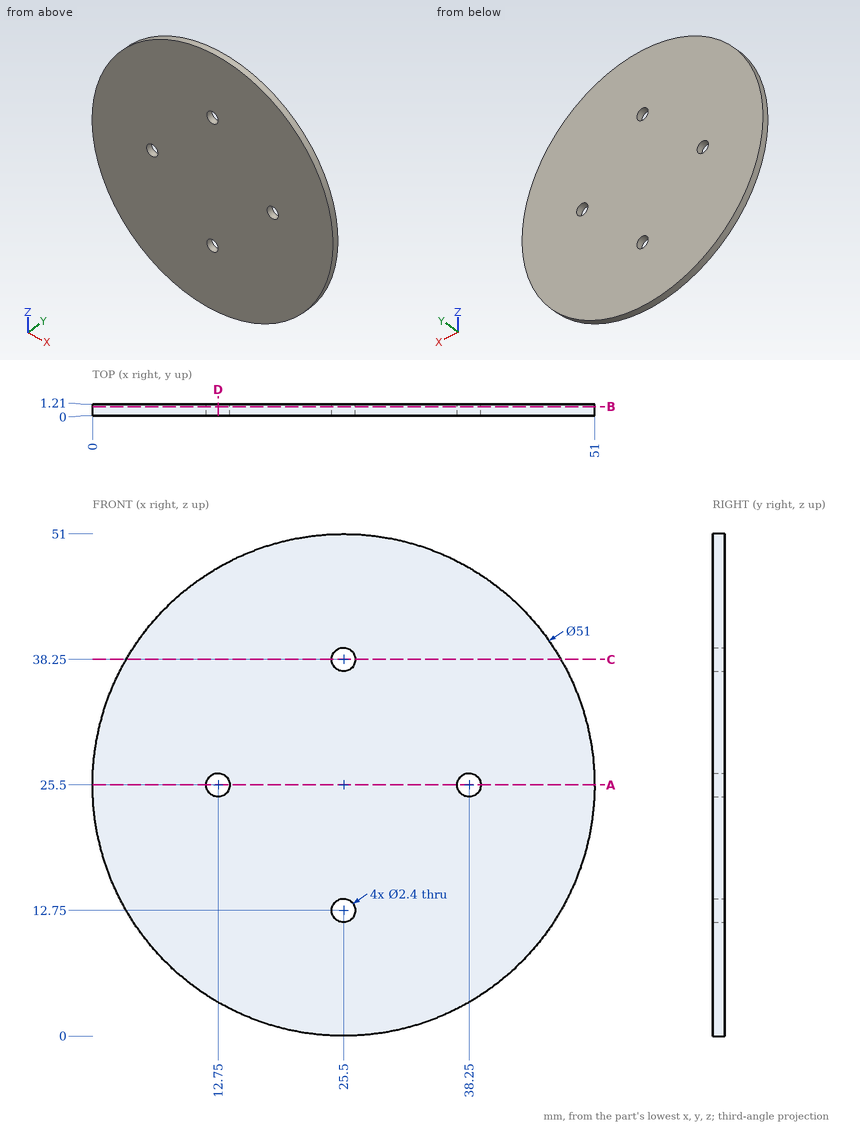
Could you check a few things on this drawing? It's one solid part, dimensions in mm from its lowest x, y, z. Coordinates: 2 decimals unless noted, no trailing zeros. Order: outer loops, then holes, each group sorted by start corner. A loop starts at its lowest first (then second) coordinate and runs counter-clockwise, first axis right, second up.
1. If we section it at D-D (x = 12.75): Please give me the cut outline in (y, z), then the cut area to 3 significant figures.
2. If we section it at C-C (z = 38.25): Please give me the cut outline in (x, y), then the cut area to 3 significant figures.
3. I need wall thicknesses on line 1 (X direction, y = 0.4, z = 25.5); line 2 (X direction, y = 1.1, z = 24.5); line 3 (X direction, y = 0.7, z = 13). Which ranges of each line are inside material? Lowest first, please.
4. If we section it at B-B (y = 0.95): Please give me the cut outline in (x, z).
5. If we section it at A-A (z = 25.5): Please give me the cut outline in (x, y), then the cut area to 3 significant figures.
Entries:
1. outline: (0, 3.42) - (1.21, 3.42) - (1.21, 24.3) - (0, 24.3) - close; (0, 26.7) - (1.21, 26.7) - (1.21, 47.58) - (0, 47.58) - close
1. area: 50.5 mm2
2. outline: (3.42, 0) - (24.3, 0) - (24.3, 1.21) - (3.42, 1.21) - close; (26.7, 0) - (47.58, 0) - (47.58, 1.21) - (26.7, 1.21) - close
2. area: 50.5 mm2
3. line 1: x = 0 to 11.55, 13.95 to 37.05, 39.45 to 51
3. line 2: x = 0.02 to 12.09, 13.41 to 37.59, 38.91 to 50.98
3. line 3: x = 3.27 to 24.33, 26.67 to 47.73
4. outline: circle Ø51 at (25.5, 25.5); hole circle Ø2.4 at (12.75, 25.5); hole circle Ø2.4 at (25.5, 12.75); hole circle Ø2.4 at (25.5, 38.25); hole circle Ø2.4 at (38.25, 25.5)
5. outline: (0, 0) - (11.55, 0) - (11.55, 1.21) - (0, 1.21) - close; (13.95, 0) - (37.05, 0) - (37.05, 1.21) - (13.95, 1.21) - close; (39.45, 0) - (51, 0) - (51, 1.21) - (39.45, 1.21) - close
5. area: 55.9 mm2
